Design review of the part shown in the three views and the two pictorial views. Dimensions are in mm from the part's minimum x, y and z. Round coordinates to 2 decimals unless told otherwise and drop trailing zeros. Order: outer loops, then holes, each group sorted by start corner. A loop starts at its lowest first (then second) coordinate and runs counter-clockwise, first axis right, second up.
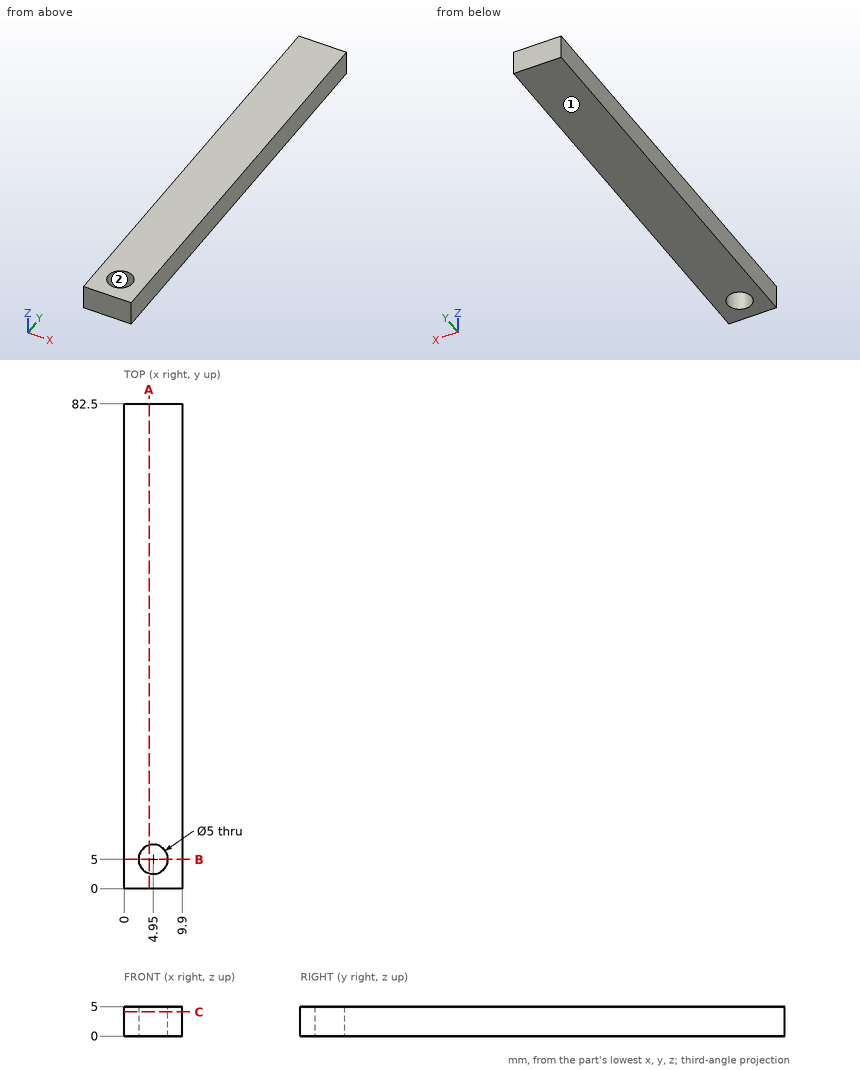
(1) Add section C-C on z = 4.1. Give the boundary of the cut face in (x, y).
(2) Draft analysis for pull direction X (two halves, no side actions). For the marked faces 1 and 2, state which applies: pulls with the +X half, pulls with the -X half, needs draft (parallel to the pull), parting line crosses it, or undercut.
(3) Add section A-A on x = 4.25. Give the boundary of the cut face in (y, z).
(4) Wall thickness on L1, parallel to Y at x = 4.95, z = 2.5; L2, parallel to Y at x = 6.5, z = 2.75: over which ranges is each line inside the solid? List them lowest first.
(5) Add section B-B on y = 5. Give the boundary of the cut face in (x, z).
Here are the results:
1. outline: (0, 0) - (9.9, 0) - (9.9, 82.5) - (0, 82.5) - close; hole circle Ø5 at (4.95, 5)
2. face 1: needs draft
2. face 2: undercut
3. outline: (0, 0) - (2.6, 0) - (2.6, 5) - (0, 5) - close; (7.4, 0) - (82.5, 0) - (82.5, 5) - (7.4, 5) - close
4. L1: y = 0 to 2.5, 7.5 to 82.5
4. L2: y = 0 to 3.04, 6.96 to 82.5
5. outline: (0, 0) - (2.45, 0) - (2.45, 5) - (0, 5) - close; (7.45, 0) - (9.9, 0) - (9.9, 5) - (7.45, 5) - close
